from build123d import *

# Parameters (mm, degrees)
F0_W     = 50.8
F0_H     = 127
F0_W_2   = 25.4
F0_H_2   = 82.55
F1_DEPTH = 15.875
F2_W     = 6.35
F2_H     = 82.55
F3_DEPTH = 6.35
F4_R     = 2.54
F5_DEPTH = 15.876
F4_R_2   = 4.0005
F6_DEPTH = 6.35


with BuildPart() as f1:
    # F0 (on Top) → F1 (new body)
    with BuildSketch(Plane.XY):
        with Locations((25.4, 63.5)):
            Rectangle(F0_W, F0_H)
        with Locations((25.4, 53.975)):
            Rectangle(F0_W_2, F0_H_2, mode=Mode.SUBTRACT)
    extrude(amount=F1_DEPTH)

    # F2 (on face) → F3 (cut)
    with BuildSketch(Plane(origin=(0, 0, 0), x_dir=(1, 0, 0), z_dir=(0, 0, -1))):
        with Locations((41.275, -53.975)):
            Rectangle(F2_W, F2_H)
        with Locations((9.525, -53.975)):
            Rectangle(F2_W, F2_H)
    extrude(amount=-F3_DEPTH, mode=Mode.SUBTRACT)

    # F4 (on face) → F5 (cut, through all)
    with BuildSketch(Plane(origin=(0, 0, 0), x_dir=(1, 0, 0), z_dir=(0, 0, -1))):
        with Locations((38.1, -114.3)):
            Circle(F4_R)
        with Locations((12.7, -114.3)):
            Circle(F4_R)
    extrude(amount=-F5_DEPTH, mode=Mode.SUBTRACT)

    # F4 (on face) → F6 (cut)
    with BuildSketch(Plane(origin=(0, 0, 0), x_dir=(1, 0, 0), z_dir=(0, 0, -1))):
        with Locations((38.1, -114.3)):
            Circle(F4_R_2)
        with Locations((38.1, -114.3)):
            Circle(F4_R, mode=Mode.SUBTRACT)
        with Locations((12.7, -114.3)):
            Circle(F4_R_2)
        with Locations((12.7, -114.3)):
            Circle(F4_R, mode=Mode.SUBTRACT)
    extrude(amount=-F6_DEPTH, mode=Mode.SUBTRACT)


solid = f1.part
Source: CAD feature listing. Evaluate the final solid. Frame: model axes, mm. A direction names the side the tool comes from. Coordinates: 2 decimals unless noted, no trailing zeros. Loops run counter-clockwise (first coordinate to the right, second up) from the corner with the lowest first, then second, coordinate; pieces in that order, holes last. Notation, with made-up numbers: (32, 18.5) -> (77, 18.5) arc R17 cw to (77, 24.5) -> close; hole circle Ø3 at (45.5, 77.5). An arc over 180 degrees is marked (long way). Answer in a Markdown table with one row per item. Add a question column.
Q1. Pull-direction query (X, two-part tool) for faces 4 (the face through (44.45, 55, 3)), 5 (the face through (50.8, 63, 8)), 6 (the face through (48, 79, 0)); classes: pulls with the +X half, pulls with the -X half, needs draft (parallel to the pull), parting line crosses it, or undercut.
Q2. Section C-C on y = 24.5. Return the cut outline in (x, z) (3 decimals), and give its area (3 significant figures).
Q3. Section A-A on z = 5. Return the cut outline in (x, y).
Q4. Reachability of faces 1 (the face through (25, 0, 8)), 2 (the face through (38.1, 53, 11)), 3 (the face through (38, 117, 6.35)) from +Z, -Z, +X, -X, +Y, -Y: full face, straight path, thin tool, end or side. Return the list, or none.
Q5. Section B-B on y = 114.3. Give the number of separate pieces and of enclosed holes in the cut face, and give its area (3 significant figures).
Q6. Ray query, line 1 along Y through (x, z) = (12.7, 4.5); line 2 along X through (y, z) = (54, 2); line 3 along X through (y, z) = (114.3, 9.25). Return the intervals inside material, ascending.
Q7. Contact query for flat-ended pins moving along their axis: pin 1 Ø5 at (y, z) = (46, 4.5) entering from -X; pin 2 Ø5 at (x, y) = (41, 39) entering from -Z. Output: stop coordinate, or through.
Computed values:
| question | item | result |
|---|---|---|
| 1 | face 4 | undercut |
| 1 | face 5 | pulls with the +X half |
| 1 | face 6 | needs draft |
| 2 | outline | (0, 0) -> (6.35, 0) -> (6.35, 6.35) -> (12.7, 6.35) -> (12.7, 15.875) -> (0, 15.875) -> close; (38.1, 6.35) -> (44.45, 6.35) -> (44.45, 0) -> (50.8, 0) -> (50.8, 15.875) -> (38.1, 15.875) -> close |
| 2 | area | 323 mm^2 |
| 3 | outline | (0, 0) -> (50.8, 0) -> (50.8, 127) -> (0, 127) -> close; hole (6.35, 12.7) -> (44.45, 12.7) -> (44.45, 95.25) -> (6.35, 95.25) -> close; hole circle Ø8 at (12.7, 114.3); hole circle Ø8 at (38.1, 114.3) |
| 4 | face 1 | +Z, -Z, +X, -X, -Y |
| 4 | face 2 | +Z, -Z |
| 4 | face 3 | -Z |
| 5 | separate pieces | 3 |
| 5 | enclosed holes | 0 |
| 5 | area | 608 mm^2 |
| 6 | line 1 | y = 0 to 12.7, 95.25 to 110.3, 118.3 to 127 |
| 6 | line 2 | x = 0 to 6.35, 44.45 to 50.8 |
| 6 | line 3 | x = 0 to 10.16, 15.24 to 35.56, 40.64 to 50.8 |
| 7 | pin 1 | stops at x = 0 |
| 7 | pin 2 | stops at z = 6.35 |
